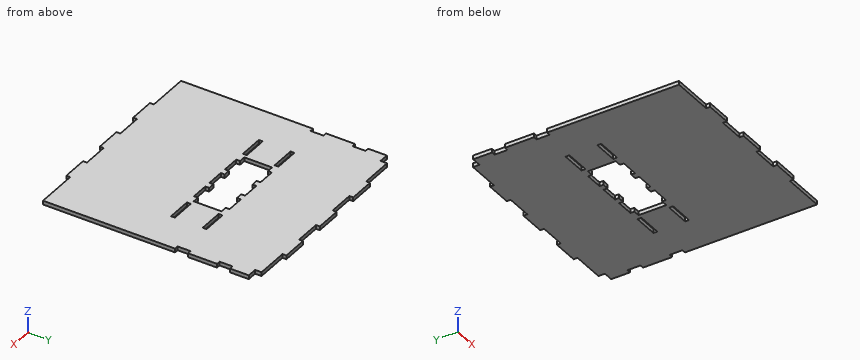
from build123d import *

# Parameters (mm, degrees)
ESQUISSE2_W                            = 330
ESQUISSE2_H                            = 340
BOSS_EXTRU_1_DEPTH                     = 6
ESQUISSE4_W                            = 65
ESQUISSE4_H                            = 6
ESQUISSE4_W_2                          = 40
ESQUISSE4_W_3                          = 6
ESQUISSE4_H_2                          = 20
ENL_V_MAT_ENCOCHE_BORD_DEPTH           = 474.852297662
ESQUISSE5_W                            = 38
ESQUISSE5_H                            = 6
ESQUISSE5_W_2                          = 15
ESQUISSE5_H_2                          = 10
ENL_V_MAT_ENCOCHE_TAGE_ROULETTES_DEPTH = 474.852297662
ENL_V_MAT_EXTRU_2_DEPTH                = 6


with BuildPart() as part:
    # Esquisse2 → Boss.-Extru.1 (new body)
    with BuildSketch(Plane.XY):
        with Locations((-165, -170)):
            Rectangle(ESQUISSE2_W, ESQUISSE2_H)
    extrude(amount=BOSS_EXTRU_1_DEPTH)

    # Esquisse4 → Enlèv. mat encoche bord (cut, through all)
    with BuildSketch(Plane(origin=(0, 0, 0), x_dir=(-1, 0, 0), z_dir=(0, 0, -1))):
        with Locations((297.5, -3)):
            Rectangle(ESQUISSE4_W, ESQUISSE4_H)
        with Locations((205, -3)):
            Rectangle(ESQUISSE4_W_2, ESQUISSE4_H)
        with Locations((125, -3)):
            Rectangle(ESQUISSE4_W_2, ESQUISSE4_H)
        with Locations((32.5, -3)):
            Rectangle(ESQUISSE4_W, ESQUISSE4_H)
        with Locations((327, -55)):
            Rectangle(ESQUISSE4_W_3, ESQUISSE4_H_2)
        with Locations((3, -55)):
            Rectangle(ESQUISSE4_W_3, ESQUISSE4_H_2)
        with Locations((297.5, -337)):
            Rectangle(ESQUISSE4_W, ESQUISSE4_H)
        with Locations((205, -337)):
            Rectangle(ESQUISSE4_W_2, ESQUISSE4_H)
        with Locations((125, -337)):
            Rectangle(ESQUISSE4_W_2, ESQUISSE4_H)
        with Locations((32.5, -337)):
            Rectangle(ESQUISSE4_W, ESQUISSE4_H)
        with Locations((327, -120)):
            Rectangle(ESQUISSE4_W_3, ESQUISSE4_H_2)
        with Locations((3, -120)):
            Rectangle(ESQUISSE4_W_3, ESQUISSE4_H_2)
    extrude(amount=-ENL_V_MAT_ENCOCHE_BORD_DEPTH, mode=Mode.SUBTRACT)

    # Esquisse5 → Enlèv. mat encoche étage + roulettes (cut, through all)
    with BuildSketch(Plane(origin=(0, 0, 0), x_dir=(-1, 0, 0), z_dir=(0, 0, -1))):
        with Locations((251, -172)):
            Rectangle(ESQUISSE5_W, ESQUISSE5_H)
        with Locations((79, -172)):
            Rectangle(ESQUISSE5_W, ESQUISSE5_H)
        with Locations((322.5, -11)):
            Rectangle(ESQUISSE5_W_2, ESQUISSE5_H_2)
        with Locations((7.5, -11)):
            Rectangle(ESQUISSE5_W_2, ESQUISSE5_H_2)
        with Locations((251, -123)):
            Rectangle(ESQUISSE5_W, ESQUISSE5_H)
        with Locations((79, -123)):
            Rectangle(ESQUISSE5_W, ESQUISSE5_H)
    extrude(amount=-ENL_V_MAT_ENCOCHE_TAGE_ROULETTES_DEPTH, mode=Mode.SUBTRACT)

    # Esquisse6 → Enlèv. mat.-Extru.2 (cut)
    with BuildSketch(Plane(origin=(0, 0, 0), x_dir=(-1, 0, 0), z_dir=(0, 0, -1))):
        Polygon((226, -169), (216, -169), (216, -175), (189, -175), (189, -169), (179, -169), (179, -175), (152, -175), (152, -169), (142, -169), (142, -175), (115, -175), (115, -169), (105, -169), (105, -126), (115, -126), (115, -120), (142, -120), (142, -126), (152, -126), (152, -120), (179, -120), (179, -126), (189, -126), (189, -120), (216, -120), (216, -126), (226, -126), align=None)
    extrude(amount=-ENL_V_MAT_EXTRU_2_DEPTH, mode=Mode.SUBTRACT)


solid = part.part
The listing builds one solid part. Answer for the finished solid, in the listing's coordinates (mm). Round coordinates to 2 decimals unless told otherwise and drop trailing zeros. Write each loop counter-clockwise with the first axis right and the second up, starting at its lowest first coordinate (ties: lowest second). Pieces come first, ordered by that corner, then holes. Notation, with made-up numbers: (69, -22) - (126, -22) arc R25 ccw to (126, 13) - close; hole circle Ø7 at (4.25, 20). An arc over 180 degrees is marked (long way). Use one line per item in the form item = value. Start each with the question number.
Item 1: A cutting plane is placed at A-A (x = -132). Write down the section's boundary in (y, z), plus the area to 3 significant figures.
Item 2: Find the intervals of material crossed by line 1 (Y direction, x = -268.5, z = 0.8); line 2 (X direction, y = -174, z = 2.3); line 3 (X direction, y = -124, z = 2.3), in increasing order. Write a range as [from, to].
Item 3: Flat-ended cylindrical pins translate along their axes: pin 1 Ø3 at (y, z) = (-3.5, 2) entering from -X; pin 2 Ø1.8 at (y, z) = (-122.5, 2.5) entering from +X. Find the tip coordinate at first contact, or state that the pin passes through.
Item 4: A cutting plane is placed at C-C (z = 4.75). Give the number of separate pieces and of enclosed holes in the cut face, plus the area to 3 significant figures.
Item 5: A cutting plane is placed at D-D (x = -295.5). Write down the section's boundary in (y, z), plus the area to 3 significant figures.
Item 6: A cutting plane is placed at B-B (x = -257). Write down the section's boundary in (y, z), plus the area to 3 significant figures.
The answers:
q1.outline = (-334, 0) - (-175, 0) - (-175, 6) - (-334, 6) - close; (-120, 0) - (-6, 0) - (-6, 6) - (-120, 6) - close
q1.area = 1,640 mm^2
q2.line_1 = [-334, -175], [-169, -126], [-120, -6]
q2.line_2 = [-330, -270], [-232, -216], [-189, -179], [-152, -142], [-115, -98], [-60, 0]
q2.line_3 = [-324, -270], [-232, -216], [-189, -179], [-152, -142], [-115, -98], [-60, -6]
q3.pin_1 = -265
q3.pin_2 = -6
q4.separate_pieces = 1
q4.enclosed_holes = 5
q4.area = 102,000 mm^2
q5.outline = (-334, 0) - (-6, 0) - (-6, 6) - (-334, 6) - close
q5.area = 1,970 mm^2
q6.outline = (-340, 0) - (-175, 0) - (-175, 6) - (-340, 6) - close; (-169, 0) - (-126, 0) - (-126, 6) - (-169, 6) - close; (-120, 0) - (0, 0) - (0, 6) - (-120, 6) - close
q6.area = 1,970 mm^2
